Autodesk Inventor part; units mm, degrees
ref_plane "YZ Plane" through (0, 0, 0) normal (1, 0, 0) x (0, 1, 0)
ref_plane "XZ Plane" through (0, 0, 0) normal (0, 1, 0) x (-1, 0, 0)
ref_plane "XY Plane" through (0, 0, 0) normal (0, 0, 1) x (1, 0, 0)
sketch "Boceto1" plane through (0, 0, 0) normal (0, 1, 0) x (-1, 0, 0)
  line L0 (0, 0) -> (0, -87) construction
  line L1 (0, 0) -> (0, 83.8978) construction
  line L2 (0, 0) -> (-87, 0) construction
  line L3 (0, 0) -> (59, 0) construction
  line L4 (-74.5, -10) -> (-49.5, -10)
  line L5 (-49.5, -10) -> (-49.5, 10)
  line L6 (-49.5, 10) -> (-74.5, 10)
  line L7 (-74.5, 10) -> (-74.5, -10)
  line L8 (-74.5, -10) -> (-49.5, 10) construction
  line L9 (-49.5, -10) -> (-74.5, 10) construction
  line L10 (-18, 63.0769) -> (-64.0145, 27.7688)
  line L11 (9, 69.9829) -> (55.0145, 34.6747)
  line L12 (9, 69.9829) -> (20.2282, 84.6157)
  line L13 (-18, 63.0769) -> (-31.752, 80.9988)
  line L14 (-64.0145, 27.7688) -> (-75.6609, 42.9467)
  line L15 (-18, -63.0769) -> (-64.0145, -27.7688)
  line L16 (9, -69.9829) -> (55.0145, -34.6747)
  line L17 (9, -69.9829) -> (20.2282, -84.6157)
  line L18 (-18, -63.0769) -> (-31.752, -80.9988)
  line L19 (-64.0145, -27.7688) -> (-75.6609, -42.9467)
  arc A0 (-75.6609, 42.9467) -> (-75.6609, -42.9467) centre (0, 0) ccw
  arc A1 (20.2282, 84.6157) -> (-31.752, 80.9988) centre (0, 0) ccw
  arc A2 (-31.752, -80.9988) -> (20.2282, -84.6157) centre (0, 0) ccw
  line L20 (59, 37.9189) -> (59, -37.9189)
  line L21 (58.0583, 38.6415) -> (59, 37.9189)
  line L22 (55.0145, 34.6747) -> (58.0583, 38.6415)
  line L23 (58.0583, -38.6415) -> (59, -37.9189)
  line L24 (55.0145, -34.6747) -> (58.0583, -38.6415)
  circle A3 centre (-15.2979, 53.8061) radius 1.55
  circle A4 centre (-55.7589, 22.7593) radius 1.55
  line L25 (-41.0072, 45.4229) -> (-35.5284, 38.2827) construction
  line L26 (-15.2979, 53.8061) -> (-55.7589, 22.7593) construction
  line L27 (32.0072, 52.3288) -> (22.9685, 40.5493) construction
  circle A5 centre (6.2979, 60.712) radius 1.55
  circle A6 centre (46.7589, 29.6652) radius 1.55
  circle A7 centre (-15.2979, -53.8061) radius 1.55
  circle A8 centre (-55.7589, -22.7593) radius 1.55
  circle A9 centre (6.2979, -60.712) radius 1.55
  circle A10 centre (46.7589, -29.6652) radius 1.55
  line L28 (46.7589, 29.6652) -> (6.2979, 60.712) construction
  point P0 (-62, 0)
  point P1 (-74.5, 0)
  point P2 (26.5284, 45.1886)
  dimension "d1" = 25
  dimension "d2" = 20
  dimension "d9" = 52.5
  dimension "d10" = 52.5
  dimension "d11" = 61
  dimension "d12" = 61
  dimension "d13" = 58
  dimension "d17" = 90
  dimension "d18" = 9
  dimension "d19" = 18
  dimension "d20" = 58
  dimension "d21" = 90
  dimension "d22" = 90
  dimension "d23" = 87
  dimension "d24" = 87
  dimension "d26" = 59
  dimension "d27" = 5
  dimension "d28" = 5
  dimension "d29" = 3.1
  dimension "d30" = 3.1
  dimension "d31" = 51
  dimension "d32" = 9
  dimension "d37" = 90
  dimension "d38" = 3.1
  dimension "d39" = 3.1
  dimension "d40" = 51
  dimension "d41" = 9
  dimension "d54" = 62
extrude "Extrusión1" add sketch "Boceto1" along normal blind 3
sketch "Boceto5" plane through (0, 3, 0) normal (0, 1, 0) x (1, 0, 0)
  arc A0 (75.6609, 42.9467) -> (75.6609, -42.9467) centre (0, 0) ccw construction
  line L0 (87, 0) -> (-107.1861, 0) construction
  line L1 (-9, -69.9829) -> (-55.0145, -34.6747)
  line L2 (-9, -69.9829) -> (5.2804, -80.9406)
  line L3 (5.2804, -80.9406) -> (0.6326, -86.9977)
  arc A1 (31.752, -80.9988) -> (-20.2282, -84.6157) centre (0, 0) ccw
  line L4 (18, -63.0769) -> (31.752, -80.9988)
  line L5 (18, -63.0769) -> (4.513, -73.4259)
  line L6 (4.513, -73.4259) -> (9.3831, -79.7727)
  line L7 (9.3831, -79.7727) -> (22.8701, -69.4238)
  line L8 (-55.0145, -34.6747) -> (-59, -31.6165)
  line L9 (-59, -37.9189) -> (-59, 37.9189)
  arc A2 (-20.2282, -84.6157) -> (31.752, -80.9988) centre (0, 0) ccw
  line L10 (18, -63.0769) -> (31.752, -80.9988)
  line L11 (64.0145, -27.7688) -> (18, -63.0769)
  line L12 (75.6609, -42.9467) -> (64.0145, -27.7688)
  arc A3 (75.6609, -42.9467) -> (75.6609, 42.9467) centre (0, 0) ccw
  line L13 (64.0145, 27.7688) -> (75.6609, 42.9467)
  line L14 (18, 63.0769) -> (64.0145, 27.7688)
  line L15 (31.752, 80.9988) -> (18, 63.0769)
  arc A4 (31.752, 80.9988) -> (-20.2282, 84.6157) centre (0, 0) ccw
  line L16 (-9, 69.9829) -> (-20.2282, 84.6157)
  line L17 (-55.0145, 34.6747) -> (-9, 69.9829)
  line L18 (-58.0583, 38.6415) -> (-55.0145, 34.6747)
  line L19 (-59, 37.9189) -> (-58.0583, 38.6415)
  line L20 (-59, -37.9189) -> (-59, 37.9189)
  line L21 (-58.0583, -38.6415) -> (-59, -37.9189)
  line L22 (-55.0145, -34.6747) -> (-58.0583, -38.6415)
  line L23 (-9, -69.9829) -> (-55.0145, -34.6747)
  line L24 (-20.2282, -84.6157) -> (-9, -69.9829)
  circle A5 centre (-46.7589, 29.6652) radius 1.55
  circle A6 centre (-6.2979, 60.712) radius 1.55
  circle A7 centre (15.2979, 53.8061) radius 1.55
  circle A8 centre (55.7589, 22.7593) radius 1.55
  circle A9 centre (-46.7589, -29.6652) radius 1.55
  circle A10 centre (-6.2979, -60.712) radius 1.55
  circle A11 centre (55.7589, -22.7593) radius 1.55
  circle A12 centre (15.2979, -53.8061) radius 1.55
  line L25 (74.5, -10) -> (74.5, 10)
  line L26 (49.5, -10) -> (74.5, -10)
  line L27 (49.5, 10) -> (49.5, -10)
  line L28 (74.5, 10) -> (49.5, 10)
  line L29 (64.0145, -27.7688) -> (18, -63.0769)
  line L30 (64.0145, -27.7688) -> (78.2949, -16.8111)
  line L31 (78.2949, -16.8111) -> (83.6749, -23.8225)
  point P0 (-55.0145, -34.6747)
  point P1 (-9, -69.9829)
  point P2 (-20.2282, -84.6157)
  point P3 (-20.2282, 84.6157)
  point P4 (31.752, -80.9988)
  point P5 (75.6609, 42.9467)
  point P6 (-20.2282, -84.6157)
  dimension "d66" = 18
  dimension "d67" = 17
  dimension "d68" = 8
  dimension "d69" = 18
extrude "Extrusión3" cut sketch "Boceto5" against normal blind 10 contours L24 A1 L16 L17 L18 L19 L9 L21 L22 L1 | L2 L3 A2 L24 | L22 L21 L9 L8 | L4 L11 L12 A1 | A1 L13 L14 L15 | L12 L30 L31 A1 | L7 L6 L5 L4
mirror "Simetría1" about plane through (0, 0, 0) normal (0, 0, 1) of "Extrusión3"
ref_plane "Plano de trabajo1" through (0, 0, 0) normal (0, 0, 1) x (1, 0, 0)
properties part number "newbaseeditado"
Here's how the part is built. I have some questions about the finished solid (model axes, mm). A direction names the side the tool comes from. Coordinates: 2 decimals unless noted, no trailing zeros. Loops run counter-clockwise (first coordinate to the right, second up) from the corner with the lowest first, then second, coordinate; pieces in that order, holes last. Notation, with made-up numbers: (-24.75, 23.25) -> (33.25, 23.25) arc R33 cw to (33.25, 51.25) -> close; hole circle Ø7 at (25, 67.5). An arc over 180 degrees is marked (long way). Use one line per item in the form item = value. Start each with the question number.
(1) Will these pins go through, and if not, where does the flat tip stop? pin 1 (1.5 mm diameter, centred on x = 25.5, y = 1, fed in from -Z); pin 2 (1 mm diameter, centred on x = 69, y = 1, fed in from -Z).
(2) If we section it at B-B (z = 47): Please give me the cut outline in (x, y).
(3) On a 3-axis mill with a long thin cutter (end or side, diameter ignored), from which of +Z, -Z, +X, -X, +Y, -Y can I reach the whole of each face in a straight line? I mean faces 1 (the face through (2.924, 1.521, -84.012)), 2 (the face through (80.95, 1.52, 20.27)), 3 (the face through (6.98, 1.52, -76.64)), 4 (the face through (27.25, 1.48, -75.13)). Say none if no direction works.
(4) We'd pull the mould along Z, two halves only. Please class faces 5 (the face through (16.03, 1.52, 74.67)), 6 (the face through (-1, 3, 1)), 7 (the face through (2.989, 1.521, 83.927)), 8 (the face through (81.023, 1.521, -20.366)): pulls with the +Z half, pulls with the -Z half, needs draft (parallel to the pull), parting line crosses it, or undercut.
(5) If we section it at D-D (y = 0.45): Give the number of separate pieces and of enclosed holes in the cut face, then the cut area to 3 significant figures.
(6) Please list where these lines run through material, in increasing order: line 1 along Z through (x, y) = (11, 1.3); line 2 along Z through (x, y) = (19, 2.45); line 3 along Z through (x, y) = (16.5, 2.8).
(7) If we section it at A-A (z = 7): Please give me the cut outline in (x, y), then the cut area to 3 significant figures.
(8) If we section it at C-C (x = -41): Please give me the cut outline in (y, z).
Verdict:
q1.pin_1 = -83.41
q1.pin_2 = -24.33
q2.outline = (-38.95, 0) -> (38.95, 0) -> (38.95, 3) -> (-38.95, 3) -> close
q3.face_1 = -X, +Y, -Y
q3.face_2 = +Z, +Y, -Y
q3.face_3 = +Y, -Y
q3.face_4 = +X, +Y, -Y
q4.face_5 = undercut
q4.face_6 = needs draft
q4.face_7 = undercut
q4.face_8 = pulls with the -Z half
q5.separate_pieces = 1
q5.enclosed_holes = 9
q5.area = 14,100 mm²
q6.line_1 = -86.3 to -78.53, -68.45 to 68.45, 78.53 to 86.3
q6.line_2 = -84.9 to -72.39, -62.31 to 62.31, 72.39 to 84.9
q6.line_3 = -85.42 to -74.31, -64.23 to -54.78, -52.83 to 52.83, 54.78 to 64.23, 74.31 to 85.42
q7.outline = (-59, 0) -> (49.5, 0) -> (49.5, 3) -> (-59, 3) -> close; (74.5, 0) -> (86.72, 0) -> (86.72, 3) -> (74.5, 3) -> close
q7.area = 362 mm²
q8.outline = (0, -45.43) -> (3, -45.43) -> (3, 45.43) -> (0, 45.43) -> close
